from build123d import *

# Parameters (mm, degrees)
SKETCH019_R      = 3.5
EXTRUDE018_DEPTH = 6
SKETCH018_W      = 25
SKETCH018_H      = 125
EXTRUDE017_DEPTH = 6
SKETCH020_R      = 3.5
EXTRUDE019_DEPTH = 6


with BuildPart() as union_parte_arriba:
    # Sketch019 → Extrude018 (new body)
    with BuildSketch(Plane.YZ):
        with BuildLine():
            ThreePointArc((82.036674, 148.659016), (70.036674, 159.65499), (58.036674, 148.659016))
            ThreePointArc((58.036674, 148.659016), (70.036674, 137.663042), (82.036674, 148.659016))
        make_face()
        with Locations((69.991982, 144.998688)):
            Circle(SKETCH019_R, mode=Mode.SUBTRACT)
    extrude(amount=EXTRUDE018_DEPTH)


with BuildPart() as union_parte_arriba_1:
    # Extrude018 placement: moved
    add(union_parte_arriba.part.moved(Location((72, 0, 0))))


with BuildPart() as palo_triangular:
    # Sketch018 → Extrude017 (new body)
    with BuildSketch(Plane.XZ):
        with Locations((84.677579, 86.042568)):
            Rectangle(SKETCH018_W, SKETCH018_H)
        Polygon((76.017071, 47.742568), (76.017071, 27.742568), (93.337579, 37.742568), align=None, mode=Mode.SUBTRACT)
        Polygon((76.017071, 53.842568), (93.337579, 43.842568), (93.337579, 63.842568), align=None, mode=Mode.SUBTRACT)
        Polygon((76.017071, 79.942568), (76.017071, 59.942568), (93.337579, 69.942568), align=None, mode=Mode.SUBTRACT)
        Polygon((76.017071, 112.142568), (76.017071, 92.142568), (93.337579, 102.142568), align=None, mode=Mode.SUBTRACT)
        Polygon((76.017071, 144.342568), (76.017071, 124.342568), (93.337579, 134.342568), align=None, mode=Mode.SUBTRACT)
        Polygon((76.017071, 86.042568), (93.337579, 96.042568), (93.337579, 76.042568), align=None, mode=Mode.SUBTRACT)
        Polygon((76.017071, 118.242568), (93.337579, 128.242568), (93.337579, 108.242568), align=None, mode=Mode.SUBTRACT)
    extrude(amount=EXTRUDE017_DEPTH)


with BuildPart() as palo_triangular_1:
    # Extrude017 placement: moved
    add(palo_triangular.part.moved(Location((0, 64, 0))))


with BuildPart() as palo_triangular001:
    # Link019 base: copy of Palo triangular
    add(palo_triangular_1.part)


with BuildPart() as palo_triangular001_1:
    # Link019 placement: moved
    add(palo_triangular001.part.moved(Location((0, 18.000008, 0))))


with BuildPart() as obj1:
    # Sketch020 → Extrude019 (new body)
    with BuildSketch(Plane.YZ):
        with BuildLine():
            ThreePointArc((57.996231, 23.111303), (69.948323, 12.063047), (81.996231, 23.006739))
            ThreePointArc((81.996231, 23.006739), (70.060056, 37.708327), (57.996231, 23.111303))
        make_face()
        with Locations((69.867134, 29.92848)):
            Circle(SKETCH020_R, mode=Mode.SUBTRACT)
    extrude(amount=EXTRUDE019_DEPTH)


with BuildPart() as obj1_1:
    # Extrude019 placement: moved
    add(obj1.part.moved(Location((91, 0, 0))))

    # Fusion023: union union parte arriba, Palo triangular001, Palo triangular
    add(union_parte_arriba_1.part)
    add(palo_triangular001_1.part)
    add(palo_triangular_1.part)


with BuildPart() as obj1_2:
    # Fusion023 placement: moved
    add(obj1_1.part.moved(Location((-10, -24, 0))))


solid = obj1_2.part
Design review of the part built by this model. Coordinates are the model's own, in mm. A direction names the side the tool comes from. Give positions to 0.01 mm unless a question says otherwise; leave off trailing zeros. Loops run counter-clockwise (first coordinate to the right, second up) from the corner with the lowest first, then second, coordinate; pieces in that order, holes last. Notation, with made-up numbers: M 72,8.5 L 78,8.5 A38 cw 78,46.5 Z; hole C -28,57.25 d1. An arc over 180 degrees is marked long. One line per question, with ' | ' between items. Start each with the question number.
1. Add section D-D (x = 70.25). Give the number of separate pieces and of enclosed holes in the cut face, plus the area to 3 significant figures.
2. Add section B-B (x = 64.5). Write out the cut boundary in (y, z), plus the area to 3 significant figures.
3. To check wall thickness, follow L1, parallel to Y at x = 85.75, z = 62; L2, parallel to X at y = 37.25, z = 20; L3, parallel to X at y = 53, z = 76. State the ranges of each line that lie inside material, in increasing order.
4. Insertion check: P1, Ø5, axis at y = 36.5, z = 50.5, coming from the -X side; P2, Ø5, axis at x = 76, y = 53.5, coming from the -Z side; P3, Ø8, axis at x = 66, z = 72.5, coming from the +Y side; P4, Ø1.5, axis at y = 40.5, z = 129, coming from the +X side. Each pin has a flat end and moves straight along its axis. Give the tip position at first contact, or say it passes through.
5. For faces 1 (the face through (64.958, 46.287, 159.652)), 2 (the face through (77, 55, 148.543)), 3 (the face through (74.8, 55.04, 107.07)), list the 3-axis set-ups (+Z, -Z, +X, -X, +Y, -Y) from which the entire face can be reached by the end or side of a thin tool; tool diameter is ignored.
6. The part is to be moulded in two halves that separate along Y. For faces 4 (the face through (66, 58, 87)), 5 (the face through (74.8, 37.04, 74.87)), 6 (the face through (66, 40, 87)), say which applies: released by +Y, released by -Y, zero draft, split by the parting line, or undercut.
7. Add section C-C (y = 44). Write out the cut boundary in (x, z), plus the area to 3 significant figures.
8. Add section A-A (z = 55.5). Write out the cut boundary in (x, y).
Worked out:
1) separate pieces: 16 | enclosed holes: 0 | area: 599 mm²
2) outline: M 34,23.54 L 40,23.54 L 40,139.28 A12.05 ccw 52,139.24 L 52,23.54 L 58,23.54 L 58,148.3 A12.05 ccw 58.04,148.66 A12.05 ccw 34.04,148.66 A12.05 ccw 34.05,148.54 L 34,148.54 Z; hole C 45.99,145 d7 | area: 1,790 mm²
3) L1: y = 34 to 40, 52 to 58 | L2: x = 81 to 87 | L3: x = 62.18 to 66.02, 72.85 to 87.18
4) P1: stops at x = 62.18 | P2: stops at z = 23.54 | P3: stops at y = 58 | P4: stops at x = 87.18
5) face 1: +Z, +X, -X | face 2: +Z, +X, +Y, -Y | face 3: +Y, -Y
6) face 4: released by +Y | face 5: zero draft | face 6: undercut
7) outline: M 62,137.84 L 68,137.84 L 68,142.12 L 62,142.12 Z; M 62,147.88 L 68,147.88 L 68,159.48 L 62,159.48 Z; M 81,12.23 L 87,12.23 L 87,26.97 L 81,26.97 Z; M 81,32.89 L 87,32.89 L 87,37.54 L 81,37.54 Z | area: 212 mm²
8) outline: M 62.18,34 L 68.89,34 L 68.89,40 L 62.18,40 Z; M 62.18,52 L 68.89,52 L 68.89,58 L 62.18,58 Z; M 83.34,34 L 87.18,34 L 87.18,40 L 83.34,40 Z; M 83.34,52 L 87.18,52 L 87.18,58 L 83.34,58 Z
